Work out the finished part from the listing and answer in its coordinate system (mm). Round coordinates to 2 decimals unless told otherwise and drop trailing zeros. Loops run counter-clockwise (first coordinate to the right, second up) from the corner with the lowest first, then second, coordinate; pieces in that order, holes last.
```python
from build123d import *

# Parameters (mm, degrees)
SKETCH_1_W          = 118.5
SKETCH_1_H          = 3
EXTRUDE_1_DEPTH     = 80
CUT_EXTRUDE_1_REACH = 145.008
SKETCH_2_R          = 1.55


with BuildPart() as part:
    # 草图1 → 凸台-拉伸1 (new body)
    with BuildSketch(Plane.XY):
        with Locations((59.25, 1.5)):
            Rectangle(SKETCH_1_W, SKETCH_1_H)
    extrude(amount=EXTRUDE_1_DEPTH)

    # 草图2 → 切除-拉伸1 (cut, up to next)
    with BuildSketch(Plane(origin=(0, 3, 0), x_dir=(1, 0, 0), z_dir=(0, 1, 0)), mode=Mode.PRIVATE) as cut_extrude_1_sk1:
        with Locations(Location((5, -10, 0), (0, 0, 270))):
            Circle(SKETCH_2_R)
    cut_extrude_1_tool1 = extrude(cut_extrude_1_sk1.sketch, amount=-CUT_EXTRUDE_1_REACH, mode=Mode.PRIVATE) & part.part
    # 草图2 → 切除-拉伸1 (cut, up to next)
    with BuildSketch(Plane(origin=(0, 3, 0), x_dir=(1, 0, 0), z_dir=(0, 1, 0)), mode=Mode.PRIVATE) as cut_extrude_1_sk2:
        with Locations(Location((5, -70, 0), (0, 0, 270))):
            Circle(SKETCH_2_R)
    cut_extrude_1_tool2 = extrude(cut_extrude_1_sk2.sketch, amount=-CUT_EXTRUDE_1_REACH, mode=Mode.PRIVATE) & part.part
    # 草图2 → 切除-拉伸1 (cut, up to next)
    with BuildSketch(Plane(origin=(0, 3, 0), x_dir=(1, 0, 0), z_dir=(0, 1, 0)), mode=Mode.PRIVATE) as cut_extrude_1_sk3:
        with Locations(Location((113.5, -70, 0), (0, 0, 270))):
            Circle(SKETCH_2_R)
    cut_extrude_1_tool3 = extrude(cut_extrude_1_sk3.sketch, amount=-CUT_EXTRUDE_1_REACH, mode=Mode.PRIVATE) & part.part
    # 草图2 → 切除-拉伸1 (cut, up to next)
    with BuildSketch(Plane(origin=(0, 3, 0), x_dir=(1, 0, 0), z_dir=(0, 1, 0)), mode=Mode.PRIVATE) as cut_extrude_1_sk4:
        with Locations(Location((113.5, -10, 0), (0, 0, 270))):
            Circle(SKETCH_2_R)
    cut_extrude_1_tool4 = extrude(cut_extrude_1_sk4.sketch, amount=-CUT_EXTRUDE_1_REACH, mode=Mode.PRIVATE) & part.part
    add(cut_extrude_1_tool1.solids().sort_by_distance((5, 3, 10))[0], mode=Mode.SUBTRACT)
    add(cut_extrude_1_tool2.solids().sort_by_distance((5, 3, 70))[0], mode=Mode.SUBTRACT)
    add(cut_extrude_1_tool3.solids().sort_by_distance((113.5, 3, 70))[0], mode=Mode.SUBTRACT)
    add(cut_extrude_1_tool4.solids().sort_by_distance((113.5, 3, 10))[0], mode=Mode.SUBTRACT)


solid = part.part
```
1. Find section B-B (z = 10). Write down the section's boundary in (x, y).
Answer key:
outline: (0, 0) - (3.45, 0) - (3.45, 3) - (0, 3) - close; (6.55, 0) - (111.95, 0) - (111.95, 3) - (6.55, 3) - close; (115.05, 0) - (118.5, 0) - (118.5, 3) - (115.05, 3) - close
2. Determine the mould class of faces 1 (the face through (111.987, 1.521, 9.664)), 2 (the face through (58, 2, 0)), 3 (the face through (0, 1, 39)) for opening direction Z: +Z half, -Z half, draft (parallel to the pull), parting line (faces both ways), or undercut.
Answer key:
face 1: undercut
face 2: -Z half
face 3: draft
3. Find section A-A (x = 113.5). Write down the section's boundary in (y, z), then the cut area to 3 significant figures.
Answer key:
outline: (0, 0) - (3, 0) - (3, 8.45) - (0, 8.45) - close; (0, 11.55) - (3, 11.55) - (3, 68.45) - (0, 68.45) - close; (0, 71.55) - (3, 71.55) - (3, 80) - (0, 80) - close
area: 221 mm2
4. Given pin 1 (2.5 mm diameter, centred on x = 5, z = 70, fed in from +Y), flat-ended and moving along its own axis, determine where the tip first touches the part or whether it passes through.
Answer key:
pin 1: passes through
5. Consider probe 1 along X at (y, z) = (1.7, 10). Determine where the line is inside the solid, lowest interval first.
Answer key:
probe 1: x = 0 to 3.45, 6.55 to 111.95, 115.05 to 118.5
